Verification items for the finished model (mm, model axes). A direction names the side the tool comes from. Round coordinates to 2 decimals unless told otherwise and drop trailing zeros. Write each loop counter-clockwise with the first axis right and the second up, starting at its lowest first coordinate (ties: lowest second). Pieces come first, ordered by that corner, then holes.
from build123d import *

# Parameters (mm, degrees)
EXTRUDE_1_DEPTH     = 3
EXTRUDE_2_DEPTH     = 10
EXTRUDE_3_DEPTH     = 3
FILLET_1_R          = 2
SKETCH_4_R          = 2.1
CUT_EXTRUDE_1_DEPTH = 37


with BuildPart() as part:
    # 草图1 → 凸台-拉伸1 (new body)
    with BuildSketch(Plane.XY):
        with BuildLine():
            Line((-12.241114452, 51.269005321), (-2.292502811, 39.48265225))
            ThreePointArc((-2.292502811, 39.48265225), (0, 38.417705443), (2.292502811, 39.48265225))
            Line((2.292502811, 39.48265225), (12.241114452, 51.269005321))
            ThreePointArc((12.241114452, 51.269005321), (15.649349314, 52.118757685), (17.528021658, 49.150806509))
            Line((17.528021658, 49.150806509), (11.493234109, -49.517097746))
            ThreePointArc((11.493234109, -49.517097746), (10.554378685, -51.519065037), (8.498829714, -52.333952128))
            Line((8.498829714, -52.333952128), (-8.498829714, -52.333952128))
            ThreePointArc((-8.498829714, -52.333952128), (-10.554378685, -51.519065037), (-11.493234109, -49.517097746))
            Line((-11.493234109, -49.517097746), (-17.528021658, 49.150806509))
            ThreePointArc((-17.528021658, 49.150806509), (-15.649349314, 52.118757685), (-12.241114452, 51.269005321))
        make_face()
    extrude(amount=EXTRUDE_1_DEPTH)

    # 草图2 → 凸台-拉伸2 (add)
    with BuildSketch(Plane.XY.offset(3)):
        with BuildLine():
            Line((-4, -52.333952128), (-4, 41.505564136))
            Line((-4, 41.505564136), (-2.292502811, 39.48265225))
            ThreePointArc((-2.292502811, 39.48265225), (0, 38.417705443), (2.292502811, 39.48265225))
            Line((2.292502811, 39.48265225), (4, 41.505564136))
            Line((4, 41.505564136), (4, -52.333952128))
            Line((4, -52.333952128), (-4, -52.333952128))
        make_face()
    extrude(amount=EXTRUDE_2_DEPTH)

    # 草图3 → 凸台-拉伸3 (add)
    with BuildSketch(Plane.XY.offset(13)):
        with BuildLine():
            Line((-12.241114452, 51.269005321), (-2.292502811, 39.48265225))
            ThreePointArc((-2.292502811, 39.48265225), (0, 38.417705443), (2.292502811, 39.48265225))
            Line((2.292502811, 39.48265225), (12.241114452, 51.269005321))
            ThreePointArc((12.241114452, 51.269005321), (15.649349314, 52.118757685), (17.528021658, 49.150806509))
            Line((17.528021658, 49.150806509), (11.493234109, -49.517097746))
            ThreePointArc((11.493234109, -49.517097746), (10.554378685, -51.519065037), (8.498829714, -52.333952128))
            Line((8.498829714, -52.333952128), (-8.498829714, -52.333952128))
            ThreePointArc((-8.498829714, -52.333952128), (-10.554378685, -51.519065037), (-11.493234109, -49.517097746))
            Line((-11.493234109, -49.517097746), (-17.528021658, 49.150806509))
            ThreePointArc((-17.528021658, 49.150806509), (-15.649349314, 52.118757685), (-12.241114452, 51.269005321))
        make_face()
    extrude(amount=EXTRUDE_3_DEPTH)

    # 圆角1
    fillet_1_edges = [part.edges().sort_by_distance(p)[0] for p in [
        (4, -5.414193996, 3),
        (-4, -5.414193996, 3),
        (4, -5.414193996, 13),
        (-4, -5.414193996, 13),
    ]]
    fillet(fillet_1_edges, radius=FILLET_1_R)

    # 草图4 → 切除-拉伸1 (cut)
    with BuildSketch(Plane.XY.offset(16)):
        with Locations((0, -42.333952128)):
            Circle(SKETCH_4_R)
        with Locations((0, 27.666047872)):
            Circle(SKETCH_4_R)
    extrude(amount=-CUT_EXTRUDE_1_DEPTH, mode=Mode.SUBTRACT)


solid = part.part
Q1. Release check for a two-part mould opening along X. For faces 4 (the flat face through (-10, 1, 3)), 5 (the flat face through (14.553, 0.508, 1.479)), 6 (the cylindrical face through (1.129, 29.437, 8.112)) record: released by +X, released by -X, zero draft, split by the parting line, or undercut.
Recorded:
face 4: zero draft
face 5: released by +X
face 6: undercut
Q2. Sectioned sample at C-C (z = 14.5). Enter the section's corners in (x, y).
Recorded:
outline: (-17.53, 49.15) - (-11.49, -49.52) arc R3 ccw to (-8.5, -52.33) - (8.5, -52.33) arc R3 ccw to (11.49, -49.52) - (17.53, 49.15) arc R3 ccw to (12.24, 51.27) - (2.29, 39.48) arc R3 cw to (-2.29, 39.48) - (-12.24, 51.27) arc R3 ccw to start; hole circle Ø4.2 at (0, -42.33); hole circle Ø4.2 at (0, 27.67)
Q3. Material ranges on line 1 along Z through (x, y) = (10, -5); line 2 along X through (y, z) = (-8, 4.75); line 3 along X through (y, z) = (47.5, 15.25), recorded low to high.
Recorded:
line 1: z = 0 to 3, 13 to 16
line 2: x = -4.02 to 4.02
line 3: x = -17.43 to -9.06, 9.06 to 17.43
Q4. Depth check by flat-ended pin: P1, Ø6.5, axis at y = -24, z = 6.5, coming from the -X side; P2, Ø6.5, axis at y = 6.5, z = 9, coming from the +X side; P3, Ø2, axis at y = 38.5, z = 7.5, coming from the +X side. Enter the tip coordinate at first touch or a pass-through.
Recorded:
P1: stops at x = -5.03
P2: stops at x = 4.44
P3: stops at x = 4
Q5. Sectioned sample at B-B (x = 7). Enter the section's corners in (y, z).
Recorded:
outline: (-52.33, 0) - (45.06, 0) - (45.06, 3) - (-52.33, 3) - close; (-52.33, 13) - (45.06, 13) - (45.06, 16) - (-52.33, 16) - close
Q6. Sectioned sample at A-A (x = 0). Enter the section's corners in (y, z), plus the area to 3 significant figures.
Recorded:
outline: (-52.33, 0) - (-44.43, 0) - (-44.43, 16) - (-52.33, 16) - close; (-40.23, 0) - (25.57, 0) - (25.57, 16) - (-40.23, 16) - close; (29.77, 0) - (38.42, 0) - (38.42, 16) - (29.77, 16) - close
area: 1,320 mm2
Q7. Tool access check on faces 1 (the cylindrical face through (10.577, -51.497, 14.479)), 2 (the cylindrical face through (-4.6, -3.56, 12.43)), 3 (the cylindrical face through (4.6, -4.9, 12.43)). Record the directions out of +Z, -Z, +X, -X, +Y, -Y that give a thin tool (end or side, any length) a straight path to the whole face; none if there is none.
Recorded:
face 1: +Z, -Z, +X, -Y
face 2: -X, +Y, -Y
face 3: +X, +Y, -Y
Q8. Sectioned sample at D-D (y = -22.5). Enter the section's corners in (x, z).
Recorded:
outline: (-13.15, 0) - (13.15, 0) - (13.15, 3) - (6, 3) arc R2 cw to (4, 5) - (4, 11) arc R2 cw to (6, 13) - (13.15, 13) - (13.15, 16) - (-13.15, 16) - (-13.15, 13) - (-6, 13) arc R2 cw to (-4, 11) - (-4, 5) arc R2 cw to (-6, 3) - (-13.15, 3) - close
